Autodesk Inventor part; units mm, degrees
ref_plane "Plan de construction1" through (115, 25, 25) normal (0, 0, -1) x (-1, 0, 0)
ref_plane "Plan YZ" through (0, 0, 0) normal (1, 0, 0) x (0, 1, 0)
ref_plane "Plan XZ" through (0, 0, 0) normal (0, 1, 0) x (-1, 0, 0)
sketch "Esquisse1" plane through (0, 0, 0) normal (0, 0, 1) x (1, 0, 0)
  arc A0 (25, 25) -> (0, 0) centre (25, 0) ccw
  line L0 (25, 25) -> (115, 25)
  arc A1 (140, 0) -> (115, 25) centre (115, 0) ccw
  line L1 (0, 0) -> (140, 0)
  dimension "d0" = 90
  dimension "d1" = 25
revolve "Révolution1" add sketch "Esquisse1" angle 180 about axis through (0, 0, 0) along (1, 0, 0)
ref_plane "Plan de construction1" through (115, 25, 25) normal (0, 0, -1) x (-1, 0, 0)
sketch "Esquisse6" plane through (115, 25, 25) normal (0, 0, -1) x (-1, 0, 0)
  line L0 (76.7668, -25) -> (78.3834, -22.2)
  line L1 (78.3834, -22.2) -> (81.6166, -22.2)
  line L2 (81.6166, -22.2) -> (83.2332, -25)
  line L3 (83.2332, -25) -> (81.6166, -27.8)
  line L4 (81.6166, -27.8) -> (78.3834, -27.8)
  line L5 (78.3834, -27.8) -> (76.7668, -25)
  line L6 (90, 0) -> (90, -50)
  line L7 (26.7668, -25) -> (28.3834, -22.2)
  line L8 (28.3834, -22.2) -> (31.6166, -22.2)
  line L9 (31.6166, -22.2) -> (33.2332, -25)
  line L10 (33.2332, -25) -> (31.6166, -27.8)
  line L11 (31.6166, -27.8) -> (28.3834, -27.8)
  line L12 (28.3834, -27.8) -> (26.7668, -25)
  line L13 (30, -25) -> (26.7668, -25) construction
  line L14 (90, -25) -> (19.1163, -25) construction
  line L15 (80, -25) -> (76.7668, -25) construction
  point P0 (115, -25)
  dimension "d4" = 5.6
  dimension "d5" = 10
  dimension "d6" = 50
  dimension "d7" = 5.6
extrude "Extrusion1" cut sketch "Esquisse6" along normal blind 12.5
sketch "Esquisse7" plane through (115, 25, 25) normal (0, 0, -1) x (-1, 0, 0)
  circle A0 centre (80, -25) radius 3.2332 construction
  circle A1 centre (30, -25) radius 3.2332 construction
  circle A2 centre (80, -25) radius 1.7
  circle A3 centre (30, -25) radius 1.7
  point P0 (115, -25)
  point P1 (78.3834, -22.2)
  point P2 (28.3834, -22.2)
  point P3 (31.6166, -27.8)
  point P4 (28.3834, -27.8)
  point P5 (81.6166, -27.8)
  point P6 (78.3834, -27.8)
  dimension "d10" = 3.4
  dimension "d11" = 3.4
extrude "Extrusion2" cut sketch "Esquisse7" along normal blind 25
sketch "Esquisse8" plane through (115, 25, 25) normal (0, 0, -1) x (-1, 0, 0)
  line L0 (0.0645, -24.9628) -> (43.3013, 0) construction
  line L1 (43.3013, 0) -> (30.8013, 21.6506) construction
  line L2 (30.8013, 21.6506) -> (-34.1506, -15.8494) construction
  line L3 (-34.1506, -15.8494) -> (-21.6506, -37.5) construction
  line L4 (-21.6506, -37.5) -> (0.0645, -24.9628) construction
  arc A0 (0, 0) -> (0, -50) centre (0, -25) ccw
  line L5 (0, 0) -> (0, -50)
  line L6 (90, 0) -> (0, 0)
  line L7 (-0.0718, -8.8756) -> (-13.0622, -16.3756) construction
  circle A1 centre (-0.0718, -8.8756) radius 1.7
  circle A2 centre (-13.0622, -16.3756) radius 1.7
  line L8 (81.6277, 0) -> (81.6277, -25) construction
  line L9 (81.6277, -25) -> (81.6277, -50) construction
  line L10 (81.6277, -25) -> (44.865, -25) construction
  line L11 (0, -50) -> (90, -50) construction
  line L12 (-34.1506, -34.1506) -> (-21.6506, -12.5) construction
  line L13 (-21.6506, -12.5) -> (0.0645, -25.0372) construction
  arc A3 (0, 0) -> (0, -50) centre (0, -25) ccw
  line L14 (0, -50) -> (0, 0)
  line L15 (-0.0718, -41.1244) -> (-13.0622, -33.6244) construction
  circle A4 centre (-0.0718, -41.1244) radius 1.7
  circle A5 centre (-13.0622, -33.6244) radius 1.7
  point P0 (115, -25)
  dimension "d14" = 60
  dimension "d15" = 14
  dimension "d16" = 18
  dimension "d17" = 33
  dimension "d18" = 3.4
  dimension "d19" = 3.4
extrude "Extrusion3" cut sketch "Esquisse8" along normal blind 25 contours A1 L5 | L5 A1 | A4 L5 | L5 A4 | A2 | A5
sketch "Esquisse9" plane through (115, 25, 25) normal (0, 0, -1) x (-1, 0, 0)
  circle A0 centre (-0.0718, -8.8756) radius 3.25
  circle A1 centre (-13.0622, -16.3756) radius 3.25
  circle A2 centre (-0.0718, -8.8756) radius 1.7
  circle A3 centre (-13.0622, -16.3756) radius 1.7
  line L0 (65.6358, 0) -> (65.6358, -25) construction
  line L1 (65.6358, -25) -> (65.6358, -50) construction
  line L2 (65.6358, -25) -> (25.9635, -25) construction
  line L3 (90, 0) -> (0, 0) construction
  line L4 (0, -50) -> (90, -50) construction
  circle A4 centre (-0.0718, -41.1244) radius 3.25
  circle A5 centre (-13.0622, -33.6244) radius 3.25
  circle A6 centre (-0.0718, -41.1244) radius 1.7
  circle A7 centre (-13.0622, -33.6244) radius 1.7
  point P0 (115, -25)
  dimension "d22" = 6.5
  dimension "d23" = 6.5
extrude "Extrusion4" cut sketch "Esquisse9" along normal blind 12.5
equation "\"d7\" = d4"
equation "\"d11\" = d10"
equation "\"d19\" = d18"
equation "\"d23\" = d22"
properties part number "P1704_004" material "PLA"
Geometry: final body of the model. Coordinates: model frame, mm. A direction names the side the tool comes from. Give positions to 0.01 mm unless a question says otherwise; leave off trailing zeros. Loops run counter-clockwise (first coordinate to the right, second up) from the corner with the lowest first, then second, coordinate; pieces in that order, holes last. Notation, with made-up numbers: (-38.75, 73) -> (-1.75, 73) arc R13 cw to (-1.75, 81) -> close; hole circle Ø6 at (-4.5, -29.5). An arc over 180 degrees is marked (long way). Put each result on its own line as item: value.
1. Pull-direction query (Y, two-part tool) for faces 3 (the cylindrical face through (70.63, 0.55, 24.994)), 4 (the cylindrical face through (126.441, -9.135, 6.337)); classes: released by +Y, released by -Y, zero draft, split by the parting line, or undercut.
Taken from the geometry:
face 3: split by the parting line
face 4: undercut
2. Set-up query: faces 1 (the flat face through (126.7, -10, 12.5)), 2 (the cylindrical face through (36.35, 1.03, 6.34)). Return all of +Z, -Z, +X, -X, +Y, -Y with unobstructed straight access to the full face (end or side cutting, diameter ignored); none if empty.
Taken from the geometry:
face 1: +Z
face 2: +Z, -Z
3. Cut plane C-C (x = 19). Return the cut outline in (y, z), plus the area to 3 significant figures.
Taken from the geometry:
outline: (-24.27, 0) -> (24.27, 0) arc R24.27 ccw to start
area: 925 mm2
4. Cut plane A-A (x = 85). Return the cut outline in (y, z), plus the area to 3 significant figures.
Taken from the geometry:
outline: (-25, 0) -> (-1.7, 0) -> (-1.7, 12.5) -> (-2.8, 12.5) -> (-2.8, 24.84) arc R25 ccw to start; (1.7, 0) -> (25, 0) arc R25 ccw to (2.8, 24.84) -> (2.8, 12.5) -> (1.7, 12.5) -> close
area: 870 mm2
5. Pin query (flat end, axial travel): P1, Ø1, axis at y = 8.5, z = 9.5, coming from the -X side; P2, Ø1.7, axis at x = 34, y = -1, coming from the +Z side; P3, Ø3, axis at x = 25, z = 10.5, coming from the +Y side. Return the tip coordinate at first contact, or that it passes through.
Taken from the geometry:
P1: stops at x = 3.21
P2: stops at z = 12.5
P3: stops at y = 23.32
6. Ray query, line 1 along X through (y, z) = (0, 5); line 2 along Z through (x, y) = (114, 1); line 3 along X through (y, z) = (18, 14.5). Return the intervals inside material, ascending. Write a range as [from, to].
Taken from the geometry:
line 1: x = [0.51, 33.3], [36.7, 83.3], [86.7, 139.49]
line 2: z = [0, 24.98]
line 3: x = [15.47, 112.42], [117.73, 124.53]
7. Cut plane B-B (z = 3.5). Return the cut outline in (x, y).
Taken from the geometry:
outline: (25, -24.75) -> (115, -24.75) arc R24.75 ccw to (115, 24.75) -> (25, 24.75) arc R24.75 ccw to start; hole circle Ø3.4 at (35, 0); hole circle Ø3.4 at (85, 0); hole circle Ø3.4 at (115.07, -16.12); hole circle Ø3.4 at (115.07, 16.12); hole circle Ø3.4 at (128.06, -8.62); hole circle Ø3.4 at (128.06, 8.62)
8. Cut plane D-D (z = 10.25). Return the cut outline in (x, y).
Taken from the geometry:
outline: (25, -22.8) -> (115, -22.8) arc R22.8 ccw to (115, 22.8) -> (25, 22.8) arc R22.8 ccw to start; hole circle Ø3.4 at (35, 0); hole circle Ø3.4 at (85, 0); hole circle Ø3.4 at (115.07, -16.12); hole circle Ø3.4 at (115.07, 16.12); hole circle Ø3.4 at (128.06, -8.62); hole circle Ø3.4 at (128.06, 8.62)
